from build123d import *

# Parameters (mm, degrees)
SZKIC1_W                      = 2
SZKIC1_H                      = 6
DODANIE_WYCI_GNI_CIE1_DEPTH   = 6
DODANIE_WYCI_GNI_CIE1_2_DEPTH = 6
SZKIC3_W                      = 6
SZKIC3_H                      = 3
DODANIE_WYCI_GNI_CIE2_DEPTH   = 5
SFAZOWANIE2_SIZE              = 6.319198065
SFAZOWANIE2_SIZE_2            = 2.3
SZKIC5_W                      = 5
SZKIC5_H                      = 3.7
SZKIC5_H_2                    = 1.091910703
WYTNIJ_WYCI_GNI_CIE1_DEPTH    = 1


with BuildPart() as part:
    # Szkic1 → Dodanie-wyci_gni_cie1 (new body)
    with BuildSketch(Plane.XY):
        with Locations((1, 3)):
            Rectangle(SZKIC1_W, SZKIC1_H)
    extrude(amount=DODANIE_WYCI_GNI_CIE1_DEPTH)



with BuildPart() as body_2:
    # Szkic1 → Dodanie-wyci_gni_cie1 2 (new body)
    with BuildSketch(Plane.XY):
        with Locations((8, 3)):
            Rectangle(SZKIC1_W, SZKIC1_H)
    extrude(amount=DODANIE_WYCI_GNI_CIE1_2_DEPTH)


with BuildPart() as part_1:
    add(part.part)

    add(body_2.part)  # Dodanie-wyci_gni_cie2 merges body 2
    # Szkic3 → Dodanie-wyci_gni_cie2 (add)
    with BuildSketch(Plane(origin=(2, 0, 0), x_dir=(0, 0, -1), z_dir=(1, 0, 0))):
        with Locations((-3, 4.5)):
            Rectangle(SZKIC3_W, SZKIC3_H)
    extrude(amount=DODANIE_WYCI_GNI_CIE2_DEPTH)

    # Sfazowanie2
    # the kernel refuses this chamfer: 6.319198065, 2.3 mm, written as the material it takes off along each edge
    with BuildSketch(Plane(origin=(-16.393230334, 6, 6), x_dir=(0, -0.9999130865277316, 0.013184058198645751), z_dir=(1, 0, 0))) as sfazowanie2_piece_1:
        Polygon((SFAZOWANIE2_SIZE * 0.999913086487, SFAZOWANIE2_SIZE * 0.0131840581981), (-SFAZOWANIE2_SIZE_2 * 0.0131840581986, SFAZOWANIE2_SIZE_2 * 0.999913086528), (0, 0), align=None)
    extrude(amount=41.786460667, mode=Mode.SUBTRACT)

    # Szkic5 → Wytnij-wyci_gni_cie1 (cut)
    with BuildSketch(Plane(origin=(0, 6, 0), x_dir=(1, 0, 0), z_dir=(0, 1, 0))):
        with Locations((4.5, -1.85)):
            Rectangle(SZKIC5_W, SZKIC5_H)
        with Locations((4.5, -4.245955352)):
            Rectangle(SZKIC5_W, SZKIC5_H_2)
    extrude(amount=-WYTNIJ_WYCI_GNI_CIE1_DEPTH, mode=Mode.SUBTRACT)


solid = part_1.part
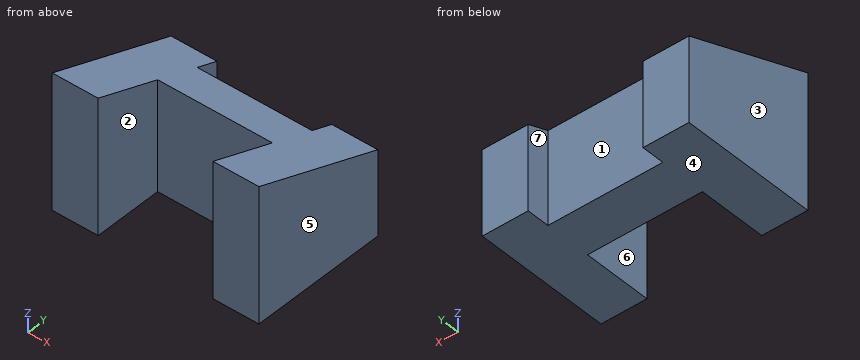
Part model, mm, in its own coordinate system. Face numbers are marked on the shaded views. A direction names the side the tool comes from. Give positions to 0.01 mm unless a question says otherwise; leave off trailing zeros. Loops run counter-clockwise (first coordinate to the right, second up) from the corner with the lowest first, then second, coordinate; pieces in that order, holes last.
(1) 3-axis set-ups, long thin cutter, end or side, ignore diameter. For the marked faces 5, 6 and 7: which of +Z, -Z, +X, -X, +Y, -Y reach the whole face in a straight line?
Return value:
face 5: +Z, -Z, +X, +Y, -Y
face 6: +Z, -Z, -Y
face 7: +Z, -Z, +Y
(2) Pin check, flat tips, straight feed: pin 1 (2.5 mm diameter, centred on x = 4.5, z = 2.5, fed in from -Y); pin 2 (3 mm diameter, centred on x = 3, y = 1.5, fed in from +Z); pin 3 (2 mm diameter, centred on x = 4.5, y = 4.5, fed in from +Z). Stop position of each tip, or through.
Return value:
pin 1: stops at y = 3
pin 2: stops at z = 5.74
pin 3: stops at z = 4.61
(3) Band-saw the part on B-B (z = 2.5). Write the cut outline in (x, y).
Return value:
outline: (0, 0) - (2, 0) - (2, 3) - (7, 3) - (7, 0) - (9, 0) - (9, 6) - (7, 6) - (7, 5) - (2, 5) - (2, 6) - (0, 6) - close
(4) Drill centre lines: line 1 along X through (y, z) = (2.05, 4.6); line 2 along Y through (x, z) = (4.5, 1.1); line 3 along Z through (x, y) = (0.5, 2.75). Where is each one in solid material? Low to high.
Return value:
line 1: x = 0 to 2, 7 to 9
line 2: y = 3 to 5
line 3: z = 0 to 4.88
(5) Band-saw the part on A-A (y = 1.05). Write the cut outline in (x, z).
Return value:
outline: (0, 0) - (2, 0) - (2, 5.5) - (0, 5.5) - close; (7, 0) - (9, 0) - (9, 5.5) - (7, 5.5) - close
(6) Band-saw the part on D-D (y = 5.25). Write the cut outline in (x, z).
Return value:
outline: (0, 0) - (2, 0) - (2, 3.97) - (0, 3.97) - close; (7, 0) - (9, 0) - (9, 3.97) - (7, 3.97) - close
(7) Pull direction X, two halves, no side cores. Call the marked faces 1, 2, 3 and 4: pulls with the +X half, pulls with the -X half, needs draft (parallel to the pull), parting line crosses it, or undercut.
Return value:
face 1: undercut
face 2: undercut
face 3: pulls with the -X half
face 4: needs draft
(8) Band-saw the part on C-C (x = 8.25). Write the cut outline in (y, z), and give its area (3 significant figures).
Return value:
outline: (0, 0) - (6, 0) - (6, 3.7) - (0, 5.88) - close
area: 28.8 mm2
